```python
from build123d import *

# Parameters (mm, degrees)
F2_DEPTH = 450
F1_W     = 580
F1_H     = 430
F3_DEPTH = 440


with BuildPart() as f2:
    # F0 (on Front) → F2 (new body)
    with BuildSketch(Plane.XZ):
        Polygon((0, 10), (-300, 10), (-300, -440), (300, -440), (300, 10), align=None)
    extrude(amount=F2_DEPTH)

    # F1 (on Front) → F3 (cut)
    with BuildSketch(Plane.XZ):
        with Locations((0, -215)):
            Rectangle(F1_W, F1_H)
    extrude(amount=F3_DEPTH, mode=Mode.SUBTRACT)


solid = f2.part
```
Can you work these out from the model? Positions are in its coordinate system, mm. A direction names the side the tool comes from. Coordinates: 2 decimals unless noted, no trailing zeros. Write each loop counter-clockwise with the first axis right and the second up, starting at its lowest first coordinate (ties: lowest second). Pieces come first, ordered by that corner, then holes. Notation, with made-up numbers: M 44,67 L 89,67 A18 ccw 89,89 Z; hole C 51.25,88.5 d9. An arc over 180 degrees is marked long. Write item = value, one per line. Start each with the question number.
Q1. Thinking about a two-plate mould opening in X: for faces 1 (the face through (290, -217, -218)), 2 (the face through (-290.3, 0, -213.9)), 3 (the face through (300, -222, -218)), which applies, released by +X, released by -X, zero draft, split by the parting line, or undercut?
Q2. If I drill on L1, parallel to Z at x = 26.5, y = -227; L2, parallel to X at y = -40, z = -116; L3, parallel to Y at x = 40, z = -13, over which ranges is the centre line in solid material (lowest first)? Write a range as [from, to].
Q3. If we section it at C-C, the plane z = -139.5: Write out the boundary of the cut face in (x, y).
Q4. On a 3-axis mill with a long thin cutter (end or side, diameter ignored), from which of +Z, -Z, +X, -X, +Y, -Y can I reach the whole of each face in a straight line? I mean faces 4 (the face through (-4, -222, -440)), 5 (the face through (-290, -217, -218)). Say none if no direction works.
Q5. I'm going to push a flat-ended pin straight in: pin 1 (2 mm diameter, centred on x = -162, z = -211, fed in from +Y). Where does the tip first touch, or does it pass through?
Q6. If we section it at B-B, the plane x = -193: Write out the boundary of the cut face in (y, z), then the cut area to 3 significant figures.
Q7. If we section it at A-A, the plane y = -359: Write out the boundary of the cut face in (x, z).
Check sheet entries:
q1.face_1 = undercut
q1.face_2 = zero draft
q1.face_3 = released by +X
q2.L1 = [-440, -430], [0, 10]
q2.L2 = [-300, -290], [290, 300]
q2.L3 = [-450, -440]
q3.outline = M -300,-450 L 300,-450 L 300,0 L 290,0 L 290,-440 L -290,-440 L -290,0 L -300,0 Z
q4.face_4 = -Z, +X, -X, +Y, -Y
q4.face_5 = +Y
q5.pin_1 = -440
q6.outline = M -450,-440 L 0,-440 L 0,-430 L -440,-430 L -440,0 L 0,0 L 0,10 L -450,10 Z
q6.area = 13,300 mm²
q7.outline = M -300,-440 L 300,-440 L 300,10 L -300,10 Z; hole M -290,-430 L 290,-430 L 290,0 L -290,0 Z
